The listing builds one solid part. Answer for the finished solid, in the listing's coordinates (mm). A direction names the side the tool comes from. Give positions to 0.01 mm unless a question says otherwise; leave off trailing zeros. Write each loop counter-clockwise with the first axis right and the second up, starting at its lowest first coordinate (ties: lowest second). Pieces come first, ordered by that corner, then holes. Notation, with made-up numbers: (17.25, 9.5) - (52.25, 9.5) arc R36 cw to (52.25, 45.5) - close; hole circle Ø5 at (12.5, 50). An arc over 180 degrees is marked (long way). Answer as CSV lines item,"result". Start each with the question number.
(1) A straight line is drawn through the part: probe 1 along X at (y, z) = (3.5, 0.95). Find the intervals that lie inside material, in ascending order.
(2) This flat-tipped pin is pushed along its axis until it touches: pin 1 Ø1.2 at (y, z) = (-3, 3.5) entering from +X. Where does it stop, or does it pass through?
(3) Find section C-C (y = 3.25). Write down the section's boundary in (x, z), then the cut area to 3 significant figures.
(4) For faces 1 (the face through (-10, -4, 3)), 2 (the face through (-1.5, 3, 2)), 3 (the face through (-1.5, -3, 2)), determine the directions among +Z, -Z, +X, -X, +Y, -Y from which every point of the face is accessible in a straight line to the end or side of a thin tool.
(5) Find section A-A (y = -2). Write down the section's boundary in (x, z).
(6) Find section B-B (z = 3.8). Write down the section's boundary in (x, y).
from build123d import *

# Parameters (mm, degrees)
F0_W     = 17.5
F0_H     = 5
F1_DEPTH = 4
F3_DEPTH = 1.5


with BuildPart() as f1:
    # F0 (on Front) → F1 (new body, symmetric)
    with BuildSketch(Plane.XZ):
        with Locations((-10.25, 2.5)):
            Rectangle(F0_W, F0_H)
    extrude(amount=F1_DEPTH, both=True)

    # F2 (on face) → F3 (join)
    with BuildSketch(Plane.YZ.offset(-1.5)):
        with BuildLine():
            ThreePointArc((0, 0), (1.767767, 0.732233), (2.5, 2.5))
            ThreePointArc((2.5, 2.5), (1.767767, 4.267767), (0, 5))
            ThreePointArc((0, 5), (-2.5, 2.5), (0, 0))
        make_face()
    extrude(amount=F3_DEPTH)


solid = f1.part
Result set:
1,probe 1,"-19 to -1.5"
2,pin 1,"x = -1.5"
3,outline,"(-19, 0) - (-1.5, 0) - (-1.5, 5) - (-19, 5) - close"
3,area,"87.5 mm^2"
4,face 1,"+Z, -Z, +X, -X, -Y"
4,face 2,"+X, +Y"
4,face 3,"+X, -Y"
5,outline,"(-19, 0) - (-1.5, 0) - (-1.5, 1) - (0, 1) - (0, 4) - (-1.5, 4) - (-1.5, 5) - (-19, 5) - close"
6,outline,"(-19, -4) - (-1.5, -4) - (-1.5, -2.14) - (0, -2.14) - (0, 2.14) - (-1.5, 2.14) - (-1.5, 4) - (-19, 4) - close"
